from build123d import *

# Parameters (mm, degrees)
SKETCH2_R          = 3
CUT_EXTRUDE1_DEPTH = 10


with BuildPart() as part:
    # Sketch1 → Revolve1 (revolve)
    with BuildSketch(Plane(origin=(0, 0, 0), x_dir=(1, 0, 0), z_dir=(0, 1, 0)), mode=Mode.PRIVATE) as revolve1_sk:
        Polygon((0, 21), (0, 31), (3, 34), (3, 45), (8, 45), (8, 34), (9.5, 34), (10, 33.5), (10, 31), (9, 31), (9, 26), (2, 26), (2, 21), align=None)
    revolve(revolve1_sk.sketch.rotate(Axis((0, 0, 0), (1, 0, 0)), 180), axis=Axis((0, 0, 0), (1, 0, 0)))

    # Sketch2 → Cut-Extrude1 (cut)
    with BuildSketch(Plane.ZY.offset(-3)):
        with Locations((0, 40)):
            Circle(SKETCH2_R)
        with Locations((34.641016151, 20)):
            Circle(SKETCH2_R)
        with Locations((34.641016151, -20)):
            Circle(SKETCH2_R)
        with Locations((0, -40)):
            Circle(SKETCH2_R)
        with Locations((-34.641016151, -20)):
            Circle(SKETCH2_R)
        with Locations((-34.641016151, 20)):
            Circle(SKETCH2_R)
    extrude(amount=-CUT_EXTRUDE1_DEPTH, mode=Mode.SUBTRACT)


solid = part.part
For this review, take the finished solid that the model builds, in its own axes (mm). A direction names the side the tool comes from. Round coordinates to 2 decimals unless told otherwise and drop trailing zeros. Loops run counter-clockwise (first coordinate to the right, second up) from the corner with the lowest first, then second, coordinate; pieces in that order, holes last. Notation, with made-up numbers: (35.25, -17) - (58.25, -17) arc R4 ccw to (58.25, -10) - close; hole circle Ø9 at (-4.75, 38.25). An arc over 180 degrees is marked (long way). Use one line per item in the form item = value.
Item 1: Consider section B-B on z = 0. State how many separate pieces and enclosed holes the cut face has, then the cut area to 3 significant figures.
Answers:
separate_pieces = 4
enclosed_holes = 0
area = 211 mm^2
Item 2: Mouldability with a two-part tool opening along Z and no side actions: class faces 1 (the flat face through (10, 30, 10)), 2 (the cylindrical face through (5.535, 39.923, 20.765)), 3 (the flat face through (2, -21.3, 1.8)) as +Z half, -Z half, draft (parallel to the pull), parting line (faces both ways), or undercut.
Answers:
face_1 = draft
face_2 = parting line
face_3 = undercut
Item 3: Consider section D-D on z = -35.5. Write out the cut boundary in (x, y), then the cut area to 3 significant figures.
Answers:
outline = (3, -27.65) - (8, -27.65) - (8, -22.87) - (3, -22.87) - close; (3, -17.13) - (8, -17.13) - (8, 17.13) - (3, 17.13) - close; (3, 22.87) - (8, 22.87) - (8, 27.65) - (3, 27.65) - close
area = 219 mm^2
Item 4: For line 1 (Y direction, x = 6.2, z = 0); line 2 (Z direction, x = 6, y = 21.5); line 3 (X direction, y = 35, z = -8.5), list the stretches that pass through material, from the lowest coordinate up.
Answers:
line_1 = -45 to -43, -37 to -26, 26 to 37, 43 to 45
line_2 = -39.53 to -37.24, -32.04 to -14.62, 14.62 to 32.04, 37.24 to 39.53
line_3 = 3 to 8
Item 5: Tool access review of faces 4 (the cylindrical face through (5.46, -21.15, -31.87)), 5 (the cylindrical face through (8.76, -33.71, -4.43)), 6 (the flat face through (3, -34, 7)): name each direction out of +Z, -Z, +X, -X, +Y, -Y from which nothing blocks a thin tool from reaching the whole face with its end or side.
Answers:
face_4 = +X, -X
face_5 = +X
face_6 = -X
Item 6: Clearance check with flat-ended pins moving along their axes: P1, Ø7, axis at y = -20, z = 34.64, coming from the -X side; P2, Ø4, axis at x = 6, z = 22, coming from the -Y side; P3, Ø6, axis at x = 5, z = -0.5, coming from the +Y side. State where each tip first meets the part, or that it passes through.
Answers:
P1 = 3
P2 = -40.31
P3 = 45
Item 7: Consider section A-A on y = 0. Write out the cut boundary in (x, z).
Answers:
outline = (0, -31) - (3, -34) - (3, -45) - (8, -45) - (8, -34) - (9.5, -34) - (10, -33.5) - (10, -31) - (9, -31) - (9, -26) - (2, -26) - (2, -21) - (0, -21) - close; (0, 21) - (2, 21) - (2, 26) - (9, 26) - (9, 31) - (10, 31) - (10, 33.5) - (9.5, 34) - (8, 34) - (8, 45) - (3, 45) - (3, 34) - (0, 31) - close
Item 8: Consider section C-C on x = 4.5. Write out the cut boundary in (y, z), then the cut area to 3 significant figures.
Answers:
outline = circle Ø90 at (0, 0); hole circle Ø6 at (-40, 0); hole circle Ø52 at (0, 0); hole circle Ø6 at (-20, -34.64); hole circle Ø6 at (-20, 34.64); hole circle Ø6 at (20, -34.64); hole circle Ø6 at (20, 34.64); hole circle Ø6 at (40, 0)
area = 4,070 mm^2
